```python
from build123d import *

# Parameters (mm, degrees)
ESQUISSE1_W             = 38.4
ESQUISSE1_H             = 18
ESQUISSE1_R             = 0.55
ESQUISSE1_R_2           = 0.582733778
BOSS_EXTRU_1_DEPTH      = 1.6
ESQUISSE2_W             = 5
ESQUISSE2_H             = 3.3
ESQUISSE2_W_2           = 4.9
ESQUISSE2_H_2           = 4.9
BOSS_EXTRU_2_DEPTH      = 1
ESQUISSE3_W             = 5
ESQUISSE3_H             = 13.2
BOSS_EXTRU_3_DEPTH      = 7
ESQUISSE4_W             = 13.2
ESQUISSE4_H             = 5.6
BOSS_EXTRU_4_DEPTH      = 9.6
CONG_2_R                = 0.5
ESQUISSE5_W             = 11.8
ESQUISSE5_H             = 4.2
ENL_V_MAT_EXTRU_1_DEPTH = 9.3
ESQUISSE6_W             = 9.8
ESQUISSE6_H             = 1.8
BOSS_EXTRU_5_DEPTH      = 8.5


with BuildPart() as part:
    # Esquisse1 → Boss.-Extru.1 (new body)
    with BuildSketch(Plane(origin=(0, 0, 0), x_dir=(1, 0, 0), z_dir=(0, 1, 0))):
        Rectangle(ESQUISSE1_W, ESQUISSE1_H)
        with Locations(Location((17.65, -7.65, 0), (0, 0, 270))):
            Circle(ESQUISSE1_R, mode=Mode.SUBTRACT)
        with Locations(Location((15.1, -7.65, 0), (0, 0, 270))):
            Circle(ESQUISSE1_R, mode=Mode.SUBTRACT)
        with Locations(Location((12.55, -7.65, 0), (0, 0, 270))):
            Circle(ESQUISSE1_R, mode=Mode.SUBTRACT)
        with Locations(Location((10, -7.65, 0), (0, 0, 270))):
            Circle(ESQUISSE1_R, mode=Mode.SUBTRACT)
        with Locations(Location((7.45, -7.65, 0), (0, 0, 270))):
            Circle(ESQUISSE1_R, mode=Mode.SUBTRACT)
        with Locations(Location((4.9, -7.65, 0), (0, 0, 270))):
            Circle(ESQUISSE1_R, mode=Mode.SUBTRACT)
        with Locations(Location((2.35, -7.65, 0), (0, 0, 270))):
            Circle(ESQUISSE1_R, mode=Mode.SUBTRACT)
        with Locations(Location((-0.2, -7.65, 0), (0, 0, 270))):
            Circle(ESQUISSE1_R, mode=Mode.SUBTRACT)
        with Locations(Location((-2.75, -7.65, 0), (0, 0, 270))):
            Circle(ESQUISSE1_R, mode=Mode.SUBTRACT)
        with Locations(Location((-5.3, -7.65, 0), (0, 0, 270))):
            Circle(ESQUISSE1_R, mode=Mode.SUBTRACT)
        with Locations(Location((-7.85, -7.65, 0), (0, 0, 270))):
            Circle(ESQUISSE1_R, mode=Mode.SUBTRACT)
        with Locations(Location((-10.4, -7.65, 0), (0, 0, 270))):
            Circle(ESQUISSE1_R, mode=Mode.SUBTRACT)
        with Locations(Location((17.65, 7.85, 0), (0, 0, 270))):
            Circle(ESQUISSE1_R, mode=Mode.SUBTRACT)
        with Locations(Location((15.1, 7.85, 0), (0, 0, 270))):
            Circle(ESQUISSE1_R, mode=Mode.SUBTRACT)
        with Locations(Location((12.55, 7.85, 0), (0, 0, 270))):
            Circle(ESQUISSE1_R, mode=Mode.SUBTRACT)
        with Locations(Location((10, 7.85, 0), (0, 0, 270))):
            Circle(ESQUISSE1_R, mode=Mode.SUBTRACT)
        with Locations(Location((7.45, 7.85, 0), (0, 0, 270))):
            Circle(ESQUISSE1_R, mode=Mode.SUBTRACT)
        with Locations(Location((4.9, 7.85, 0), (0, 0, 270))):
            Circle(ESQUISSE1_R, mode=Mode.SUBTRACT)
        with Locations(Location((2.35, 7.85, 0), (0, 0, 270))):
            Circle(ESQUISSE1_R, mode=Mode.SUBTRACT)
        with Locations(Location((-0.2, 7.85, 0), (0, 0, 270))):
            Circle(ESQUISSE1_R, mode=Mode.SUBTRACT)
        with Locations(Location((-2.75, 7.85, 0), (0, 0, 270))):
            Circle(ESQUISSE1_R, mode=Mode.SUBTRACT)
        with Locations(Location((-5.3, 7.85, 0), (0, 0, 270))):
            Circle(ESQUISSE1_R, mode=Mode.SUBTRACT)
        with Locations(Location((-7.85, 7.85, 0), (0, 0, 270))):
            Circle(ESQUISSE1_R, mode=Mode.SUBTRACT)
        with Locations(Location((-10.4, 7.85, 0), (0, 0, 270))):
            Circle(ESQUISSE1_R, mode=Mode.SUBTRACT)
        with Locations(Location((17.65, -4.617266222, 0), (0, 0, 270))):
            Circle(ESQUISSE1_R_2, mode=Mode.SUBTRACT)
        with Locations(Location((17.65, -1.584532444, 0), (0, 0, 270))):
            Circle(ESQUISSE1_R, mode=Mode.SUBTRACT)
        with Locations(Location((17.65, 5.35, 0), (0, 0, 270))):
            Circle(ESQUISSE1_R, mode=Mode.SUBTRACT)
        with Locations(Location((17.65, 2.85, 0), (0, 0, 270))):
            Circle(ESQUISSE1_R, mode=Mode.SUBTRACT)
        with Locations(Location((15.1, -4.617266222, 0), (0, 0, 270))):
            Circle(ESQUISSE1_R_2, mode=Mode.SUBTRACT)
        with Locations(Location((12.55, -4.617266222, 0), (0, 0, 270))):
            Circle(ESQUISSE1_R_2, mode=Mode.SUBTRACT)
        with Locations(Location((10, -4.617266222, 0), (0, 0, 270))):
            Circle(ESQUISSE1_R_2, mode=Mode.SUBTRACT)
        with Locations(Location((15.1, -1.584532444, 0), (0, 0, 270))):
            Circle(ESQUISSE1_R, mode=Mode.SUBTRACT)
        with Locations(Location((12.55, -1.584532444, 0), (0, 0, 270))):
            Circle(ESQUISSE1_R, mode=Mode.SUBTRACT)
        with Locations(Location((10, -1.584532444, 0), (0, 0, 270))):
            Circle(ESQUISSE1_R, mode=Mode.SUBTRACT)
        with Locations(Location((15.1, 5.35, 0), (0, 0, 270))):
            Circle(ESQUISSE1_R, mode=Mode.SUBTRACT)
        with Locations(Location((15.1, 2.85, 0), (0, 0, 270))):
            Circle(ESQUISSE1_R, mode=Mode.SUBTRACT)
        with Locations(Location((12.55, 5.35, 0), (0, 0, 270))):
            Circle(ESQUISSE1_R, mode=Mode.SUBTRACT)
        with Locations(Location((12.55, 2.85, 0), (0, 0, 270))):
            Circle(ESQUISSE1_R, mode=Mode.SUBTRACT)
        with Locations(Location((10, 5.35, 0), (0, 0, 270))):
            Circle(ESQUISSE1_R, mode=Mode.SUBTRACT)
        with Locations(Location((10, 2.85, 0), (0, 0, 270))):
            Circle(ESQUISSE1_R, mode=Mode.SUBTRACT)
        with Locations(Location((-10.4, 5.35, 0), (0, 0, 270))):
            Circle(ESQUISSE1_R, mode=Mode.SUBTRACT)
        with Locations(Location((-7.85, 5.35, 0), (0, 0, 270))):
            Circle(ESQUISSE1_R, mode=Mode.SUBTRACT)
        with Locations(Location((-5.3, 5.35, 0), (0, 0, 270))):
            Circle(ESQUISSE1_R, mode=Mode.SUBTRACT)
        with Locations(Location((-2.75, 5.35, 0), (0, 0, 270))):
            Circle(ESQUISSE1_R, mode=Mode.SUBTRACT)
        with Locations(Location((-0.2, 5.35, 0), (0, 0, 270))):
            Circle(ESQUISSE1_R, mode=Mode.SUBTRACT)
    extrude(amount=BOSS_EXTRU_1_DEPTH)

    # Esquisse2 → Boss.-Extru.2 (add)
    with BuildSketch(Plane(origin=(0, 1.6, 0), x_dir=(1, 0, 0), z_dir=(0, 1, 0))):
        with Locations((-5.7, -4.35)):
            Rectangle(ESQUISSE2_W, ESQUISSE2_H)
        with Locations((1.75, 0)):
            Rectangle(ESQUISSE2_W_2, ESQUISSE2_H_2)
    extrude(amount=BOSS_EXTRU_2_DEPTH)

    # Esquisse3 → Boss.-Extru.3 (add)
    with BuildSketch(Plane(origin=(0, 1.6, 0), x_dir=(1, 0, 0), z_dir=(0, 1, 0))):
        with Locations((-14.7, 0)):
            Rectangle(ESQUISSE3_W, ESQUISSE3_H)
    extrude(amount=BOSS_EXTRU_3_DEPTH)

    # Esquisse4 → Boss.-Extru.4 (add)
    with BuildSketch(Plane.ZY.offset(17.2)):
        with Locations((0, 5.8)):
            Rectangle(ESQUISSE4_W, ESQUISSE4_H)
    extrude(amount=BOSS_EXTRU_4_DEPTH)

    # Congé2
    cong_2_edges = [part.edges().sort_by_distance(p)[0] for p in [
        (-12.2, 5.1, 6.6),
        (-12.2, 5.1, -6.6),
        (-12.2, 8.6, 0),
        (-19.5, 8.6, -6.6),
        (-19.5, 8.6, 6.6),
        (-17.2, 2.3, 6.6),
        (-17.2, 2.3, -6.6),
        (-17.2, 3, 0),
        (-22, 3, -6.6),
        (-22, 3, 6.6),
    ]]
    fillet(cong_2_edges, radius=CONG_2_R)

    # Esquisse5 → Enlèv. mat.-Extru.1 (cut)
    with BuildSketch(Plane.ZY.offset(26.8)):
        with Locations((0, 5.8)):
            Rectangle(ESQUISSE5_W, ESQUISSE5_H)
    extrude(amount=-ENL_V_MAT_EXTRU_1_DEPTH, mode=Mode.SUBTRACT)

    # Esquisse6 → Boss.-Extru.5 (add)
    with BuildSketch(Plane.ZY.offset(17.5)):
        with Locations((0, 6.4)):
            Rectangle(ESQUISSE6_W, ESQUISSE6_H)
    extrude(amount=BOSS_EXTRU_5_DEPTH)


solid = part.part
```
For this review, take the finished solid that the model builds, in its own axes (mm). A direction names the side the tool comes from. Give positions to 0.01 mm unless a question says otherwise; leave off trailing zeros. Write each loop counter-clockwise with the first axis right and the second up, starting at its lowest first coordinate (ties: lowest second). Pieces come first, ordered by that corner, then holes. Notation, with made-up numbers: M -18,3.25 L 8,3.25 A25 cw 8,18.25 Z; hole C -20.5,13 d10. An arc over 180 degrees is marked long. One line per item, written item: value.
1) For P1, Ø5, axis at x = 13, z = 5, coming from the +Y side; P2, Ø0.7, axis at x = 4.9, z = 7.65, coming from the +Y side; P3, Ø4, axis at y = 6.5, z = 5.5, coming from the +X side; P4, Ø0.7, axis at y = 2, z = -2.5, coming from the -X side, all flat-tipped, find the tip position at first contact; note any pin that passes through.
Results are:
P1: stops at y = 1.6
P2: passes through
P3: stops at x = -12.2
P4: stops at x = -17.2
2) For faces 4 (the flat face through (-20, 6, 6.6)), 5 (the flat face through (-3.2, 2, 4)), 6 (the flat face through (-22, 7.3, 0)), 7 (the cylindrical face through (-2.585, 0.789, -7.325)), list the 3-axis set-ups (+Z, -Z, +X, -X, +Y, -Y) from which the entire face can be reached by the end or side of a thin tool; tool diameter is ignored.
Results are:
face 4: +Z, +X, -X, +Y
face 5: +Z, -Z, +X, +Y
face 6: -X
face 7: +Y, -Y
3) Take a section at B-B, the plane x = 7.45. Write out the cut boundary in (y, z).
Results are:
outline: M 0,-9 L 1.6,-9 L 1.6,-8.4 L 0,-8.4 Z; M 0,-7.3 L 1.6,-7.3 L 1.6,7.1 L 0,7.1 Z; M 0,8.2 L 1.6,8.2 L 1.6,9 L 0,9 Z
4) Take a section at D-D, the plane x = -14. Write out the cut boundary in (y, z), then the cut area to 3 significant figures.
Results are:
outline: M 0,-9 L 1.6,-9 L 1.6,-6.6 L 8.1,-6.6 A0.5 ccw 8.6,-6.1 L 8.6,6.1 A0.5 ccw 8.1,6.6 L 1.6,6.6 L 1.6,9 L 0,9 Z
area: 121 mm²
5) For line 1 (Y direction, x = -19.5, z = 4.75); line 2 (Z direction, x = -18, y = 8); line 3 (Y direction, x = 1.5, z = -4), list the stretches that pass through material, from the lowest coordinate up. Write a range as from..to.
Results are:
line 1: y = 3..3.7, 5.5..7.3, 7.9..8.6
line 2: z = -6.6..6.6
line 3: y = 0..1.6
6) Take a section at A-A, the plane x = 15.1. Write out the cut boundary in (y, z), then the cut area to 3 significant figures.
Results are:
outline: M 0,-9 L 1.6,-9 L 1.6,-8.4 L 0,-8.4 Z; M 0,-7.3 L 1.6,-7.3 L 1.6,-5.9 L 0,-5.9 Z; M 0,-4.8 L 1.6,-4.8 L 1.6,-3.4 L 0,-3.4 Z; M 0,-2.3 L 1.6,-2.3 L 1.6,1.03 L 0,1.03 Z; M 0,2.13 L 1.6,2.13 L 1.6,4.03 L 0,4.03 Z; M 0,5.2 L 1.6,5.2 L 1.6,7.1 L 0,7.1 Z; M 0,8.2 L 1.6,8.2 L 1.6,9 L 0,9 Z
area: 18.1 mm²
7) Take a section at C-C, the plane z = -4.25. Write out the cut boundary in (x, y), then the cut area to 3 significant figures.
Results are:
outline: M -26.8,3 L -17.7,3 A0.5 cw -17.2,2.5 L -17.2,1.6 L -19.2,1.6 L -19.2,0 L 19.2,0 L 19.2,1.6 L -12.2,1.6 L -12.2,8.1 A0.5 ccw -12.7,8.6 L -26.8,8.6 L -26.8,7.9 L -17.5,7.9 L -17.5,7.3 L -26,7.3 L -26,5.5 L -17.5,5.5 L -17.5,3.7 L -26.8,3.7 Z
area: 126 mm²
8) The part is to be moulded in two halves that separate along X. For faces 1 (the flat face through (4.2, 2, 0)), 2 (the cylindrical face through (2.515, 0.789, 8.175)), 3 (the flat face through (-20, 8.6, 0)), say which applies: +X half, -X half, draft (parallel to the pull), parting line (faces both ways), or undercut.
Results are:
face 1: +X half
face 2: undercut
face 3: draft
